```python
from build123d import *

# Parameters (mm, degrees)
SKETCH1_R           = 63.5
BOSS_EXTRUDE1_DEPTH = 38.1
CUT_EXTRUDE2_DEPTH  = 31.75


with BuildPart() as part:
    # Sketch1 → Boss-Extrude1 (new body)
    with BuildSketch(Plane(origin=(0, 0, 0), x_dir=(1, 0, 0), z_dir=(0, 1, 0))):
        with Locations(Location((0, 0, 0), (0, 0, 90))):
            Circle(SKETCH1_R)
    extrude(amount=BOSS_EXTRUDE1_DEPTH)

    # Sketch2 → Cut-Extrude2 (cut)
    with BuildSketch(Plane(origin=(0, 38.1, 0), x_dir=(1, 0, 0), z_dir=(0, 1, 0))):
        with BuildLine():
            Line((-1.7819572, -9.111319007), (-16.057301334, -50.738697991))
            ThreePointArc((-16.057301334, -50.738697991), (-15.89484722, -52.75977688), (-14.304875125, -54.018005773))
            ThreePointArc((-14.304875125, -54.018005773), (3.484226214, -55.771270092), (20.916794468, -51.817584942))
            ThreePointArc((20.916794468, -51.817584942), (22.337802979, -50.371249564), (22.247447967, -48.345666393))
            Line((22.247447967, -48.345666393), (2.902107489, -8.818689111))
            ThreePointArc((2.902107489, -8.818689111), (0.462316687, -7.400205158), (-1.7819572, -9.111319007))
        make_face()
        with BuildLine():
            Line((8.704163204, -3.229403726), (51.669220951, -12.749274735))
            ThreePointArc((51.669220951, -12.749274735), (53.309221074, -13.941562792), (53.554027291, -15.954327341))
            ThreePointArc((53.554027291, -15.954327341), (45.776114287, -32.048740393), (33.314033776, -44.863677441))
            ThreePointArc((33.314033776, -44.863677441), (31.338979429, -45.322274799), (29.657547842, -44.189164464))
            Line((29.657547842, -44.189164464), (6.012483905, -7.074004722))
            ThreePointArc((6.012483905, -7.074004722), (6.073963109, -4.252498707), (8.704163204, -3.229403726))
        make_face()
        with BuildLine():
            Line((7.951806494, 4.791688532), (42.1830167, 32.447580836))
            ThreePointArc((42.1830167, 32.447580836), (44.13770839, 32.986405118), (45.863985261, 31.922864157))
            ThreePointArc((45.863985261, 31.922864157), (53.597654639, 15.807144497), (55.846795761, -1.926084944))
            ThreePointArc((55.846795761, -1.926084944), (54.973915369, -3.756175388), (53.039658589, -4.3642888))
            Line((53.039658589, -4.3642888), (9.279401997, 0.290179402))
            ThreePointArc((9.279401997, 0.290179402), (7.111791423, 2.097426005), (7.951806494, 4.791688532))
        make_face()
        with BuildLine():
            Line((1.211577307, 9.204541593), (0.932140496, 53.210746228))
            ThreePointArc((0.932140496, 53.210746228), (1.729601044, 55.074937175), (3.637426875, 55.761487836))
            ThreePointArc((3.637426875, 55.761487836), (21.059067856, 51.759927174), (36.325781471, 42.461888801))
            ThreePointArc((36.325781471, 42.461888801), (37.212371773, 40.638400701), (36.481824607, 38.746985345))
            Line((36.481824607, 38.746985345), (5.55874112, 7.435852518))
            ThreePointArc((5.55874112, 7.435852518), (2.794295742, 6.867946156), (1.211577307, 9.204541593))
        make_face()
        with BuildLine():
            Line((-6.440994304, 6.686187096), (-41.020656513, 33.905134408))
            ThreePointArc((-41.020656513, 33.905134408), (-41.980931166, 35.690918215), (-41.328188139, 37.610573848))
            ThreePointArc((-41.328188139, 37.610573848), (-27.33742655, 48.736428979), (-10.549287178, 54.875194214))
            ThreePointArc((-10.549287178, 54.875194214), (-8.570846762, 54.431432191), (-7.547567398, 52.680989231))
            Line((-7.547567398, 52.680989231), (-2.347765198, 8.982177024))
            ThreePointArc((-2.347765198, 8.982177024), (-3.627361626, 6.466762771), (-6.440994304, 6.686187096))
        make_face()
        with BuildLine():
            Line((-9.243365832, -0.867002658), (-52.084062499, -10.931735159))
            ThreePointArc((-52.084062499, -10.931735159), (-54.078965953, -10.569090123), (-55.172834542, -8.861869364))
            ThreePointArc((-55.172834542, -8.861869364), (-55.148281182, 9.013405721), (-49.480527415, 25.966359134))
            ThreePointArc((-49.480527415, 25.966359134), (-47.900042872, 27.236485042), (-45.89348721, 26.94513373))
            Line((-45.89348721, 26.94513373), (-8.486356436, 3.764739028))
            ThreePointArc((-8.486356436, 3.764739028), (-7.317541705, 1.195975121), (-9.243365832, -0.867002658))
        make_face()
        with BuildLine():
            Line((-5.085294358, -7.767321727), (-23.927107102, -47.536785185))
            ThreePointArc((-23.927107102, -47.536785185), (-25.454436367, -48.870358028), (-27.471211214, -48.661144195))
            ThreePointArc((-27.471211214, -48.661144195), (-41.431355264, -37.496895885), (-51.15192129, -22.495673991))
            ThreePointArc((-51.15192129, -22.495673991), (-51.159529717, -20.468090867), (-49.680675096, -19.080957051))
            Line((-49.680675096, -19.080957051), (-8.234548188, -4.287624243))
            ThreePointArc((-8.234548188, -4.287624243), (-5.49746363, -4.975406188), (-5.085294358, -7.767321727))
        make_face()
    extrude(amount=-CUT_EXTRUDE2_DEPTH, mode=Mode.SUBTRACT)


solid = part.part
```
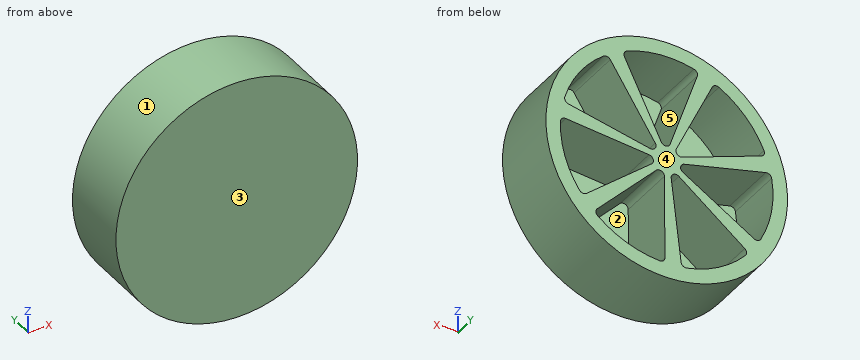
Here's how the part is built. I have some questions about the finished solid (model axes, mm). Face numbers are marked on the shaded views. A direction names the side the tool comes from. Give positions to 0.01 mm unless a question says otherwise; leave off trailing zeros. Write each loop counter-clockwise with the first axis right and the second up, starting at its lowest first coordinate (ties: lowest second). Pieces come first, ordered by that corner, then holes.
(1) On a 3-axis mill with a long thin cutter (end or side, diameter ignored), from which of +Z, -Z, +X, -X, +Y, -Y can I reach the whole of each face in a straight line? I mean the marked faces 4 and 5. Say none if no direction works.
Output values:
face 4: +Z, -Z, +X, -X, +Y
face 5: +Y
(2) If I drill on L1, parallel to Z at x = -51, y = 35; L2, parallel to X at y = 13.5, z = 44; L3, parallel to X at y = 26.5, z = -17, over which ranges is the centre line in solid material (lowest first)?
Output values:
L1: z = -37.83 to -22.84, 10.68 to 20.16, 22.84 to 37.83
L2: x = -45.78 to -34.45, -22.25 to -13.75, 20.12 to 29.54, 34.45 to 45.78
L3: x = -61.18 to -53.23, -29.84 to -19.54, -3.3 to 1.16, 15 to 23.06, 53.23 to 61.18
(3) Imagine slicing it at C-C, the plane x = -30. Write out the boundary of the cut face in (y, z), and give its area (3 significant figures).
Output values:
outline: (0, -55.97) - (38.1, -55.97) - (38.1, -47.14) - (6.35, -47.14) - (6.35, -25.23) - (38.1, -25.23) - (38.1, -17.1) - (6.35, -17.1) - (6.35, 5.74) - (38.1, 5.74) - (38.1, 12.06) - (6.35, 12.06) - (6.35, 47.14) - (38.1, 47.14) - (38.1, 55.97) - (0, 55.97) - close
area: 1,730 mm2
(4) Imagine slicing it at D-D, the plane x = 13.5. Write out the boundary of the cut face in (y, z), and give its area (3 significant figures).
Output values:
outline: (0, -62.05) - (38.1, -62.05) - (38.1, -54.22) - (6.35, -54.22) - (6.35, -15.48) - (38.1, -15.48) - (38.1, -9.27) - (6.35, -9.27) - (6.35, 0.16) - (38.1, 0.16) - (38.1, 4.29) - (6.35, 4.29) - (6.35, 18.83) - (38.1, 18.83) - (38.1, 30.47) - (6.35, 30.47) - (6.35, 54.22) - (38.1, 54.22) - (38.1, 62.05) - (0, 62.05) - close
area: 1,980 mm2
(5) Will these pins go through, and if not, where does the flat tip stop? pin 1 (5 mm diameter, centred on y = 12, z = 30.5, fed in from +X); pin 2 (2 mm diameter, centred on y = 29, z = 40.5, fed in from -X); pin 3 (3 mm diameter, centred on x = -25, y = 34, fed in from +Z).
Output values:
pin 1: stops at x = 56.99
pin 2: stops at x = -49.72
pin 3: stops at z = 58.99
(6) Imagine slicing it at B-B, the plane y = 24. Count the separate pieces of the cut face and the enclosed holes in it, and give its area (3 significant figures).
Output values:
separate pieces: 1
enclosed holes: 7
area: 5,130 mm2
(7) Imagine slicing it at A-A, the plane z = -12.5. Write out the boundary of the cut face in (x, y).
Output values:
outline: (-62.26, 0) - (62.26, 0) - (62.26, 38.1) - (54.46, 38.1) - (54.46, 6.35) - (17.49, 6.35) - (17.49, 38.1) - (10.56, 38.1) - (10.56, 6.35) - (1.19, 6.35) - (1.19, 38.1) - (-2.77, 38.1) - (-2.77, 6.35) - (-13.83, 6.35) - (-13.83, 38.1) - (-22.58, 38.1) - (-22.58, 6.35) - (-54.46, 6.35) - (-54.46, 38.1) - (-62.26, 38.1) - close
(8) Thinking about a two-plate mould opening in Z: for the marked faces 1, 2 and 3, which applies, pulls with the +Z half, pulls with the -Z half, needs draft (parallel to the pull), parting line crosses it, or undercut?
Output values:
face 1: parting line crosses it
face 2: undercut
face 3: needs draft
